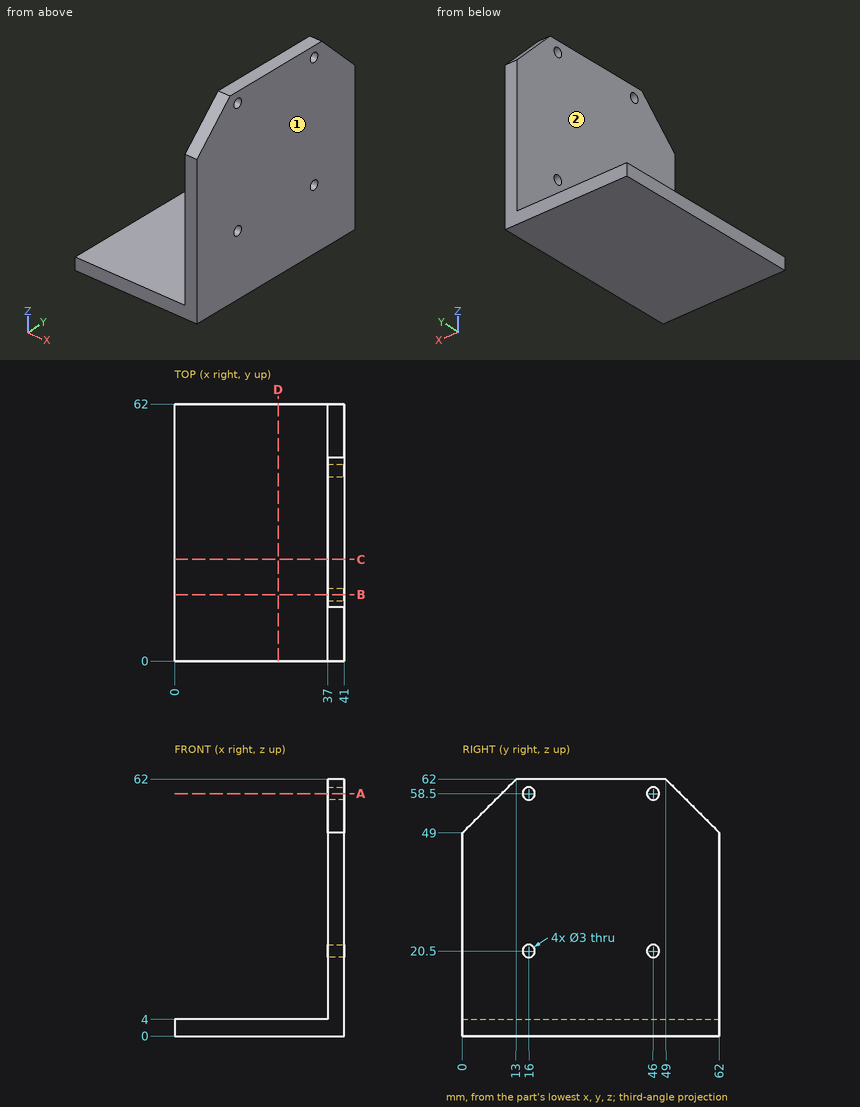
Geometry: see drawing. Coordinates: mm, zero at the bounding-box minimum. A direction names the side the tool comes from. Round coordinates to 2 decimals unless told otherwise and drop trailing zeros. Loops run counter-clockwise (first coordinate to the right, second up) from the corner with the lowest first, then second, coordinate; pieces in that order, holes last. Notation, with made-up numbers: (76, 61.5) -> (120, 61.5) arc R29 cw to (120, 83.5) -> close; hole circle Ø5 at (-2.5, 29.25). An arc over 180 degrees is marked (long way). Use one line per item in the form item = value. Start each with the question number.
Item 1: Material intervals for L1, parallel to Y at x = 39.6, z = 20.5; L2, parallel to Y at x = 39, z = 20; L3, parallel to X at y = 19, z = 48.5, sorted ascending. Write a range as from..to.
Item 2: Contact query for flat-ended pins moving along their axis: pin 1 Ø12 at (y, z) = (31.5, 11.5) entering from -X; pin 2 Ø1.5 at (x, y) = (20, 9) entering from +Z. Output: stop coordinate, or through.
Item 3: Section query A-A on z = 58.5. Return the cut outline in (x, y), then the cut area to 3 significant figures.
Item 4: Section query B-B on y = 16. Return the cut outline in (x, z).
Item 5: Set-up query: the marked faces 1 and 2. Return all of +Z, -Z, +X, -X, +Y, -Y with unobstructed straight access to the full face (end or side cutting, diameter ignored); none if empty.
Item 6: Section query C-C on y = 24.5. Return the cut outline in (x, z).
Item 7: Section query D-D on x = 25. Return the cut outline in (y, z).
Ans:
q1.L1 = 0..14.5, 17.5..44.5, 47.5..62
q1.L2 = 0..14.59, 17.41..44.59, 47.41..62
q1.L3 = 37..41
q2.pin_1 = 37
q2.pin_2 = 4
q3.outline = (37, 9.5) -> (41, 9.5) -> (41, 14.5) -> (37, 14.5) -> close; (37, 17.5) -> (41, 17.5) -> (41, 44.5) -> (37, 44.5) -> close; (37, 47.5) -> (41, 47.5) -> (41, 52.5) -> (37, 52.5) -> close
q3.area = 148 mm^2
q4.outline = (0, 0) -> (41, 0) -> (41, 19) -> (37, 19) -> (37, 4) -> (0, 4) -> close; (37, 22) -> (41, 22) -> (41, 57) -> (37, 57) -> close; (37, 60) -> (41, 60) -> (41, 62) -> (37, 62) -> close
q5.face_1 = +Z, -Z, +X, +Y, -Y
q5.face_2 = +Z, -X, +Y, -Y
q6.outline = (0, 0) -> (41, 0) -> (41, 62) -> (37, 62) -> (37, 4) -> (0, 4) -> close
q7.outline = (0, 0) -> (62, 0) -> (62, 4) -> (0, 4) -> close
